Autodesk Inventor part; units mm, degrees
ref_plane "YZ Plane" through (0, 0, 0) normal (1, 0, 0) x (0, 1, 0)
ref_plane "XZ Plane" through (0, 0, 0) normal (0, 1, 0) x (-1, 0, 0)
ref_plane "XY Plane" through (0, 0, 0) normal (0, 0, 1) x (1, 0, 0)
sketch "Sketch1" plane through (0, 0, 0) normal (0, 1, 0) x (-1, 0, 0)
  line L0 (0, 0) -> (115, 0)
  line L1 (115, 0) -> (115, -215)
  line L2 (115, -215) -> (0, -215)
  line L3 (0, -215) -> (0, 0)
  dimension "d0" = 115
  dimension "d1" = 215
extrude "Extrusion1" add sketch "Sketch1" along normal blind 50
sketch "Sketch2" plane through (-115, 0, 0) normal (0, 0, 1) x (1, 0, 0)
  line L0 (115, 0) -> (115, 5)
  line L1 (115, 0) -> (115, 50)
  line L2 (115, 5) -> (43, 5)
  line L3 (43, 5) -> (43, 17)
  line L4 (43, 17) -> (115, 17)
  line L5 (115, 17) -> (115, 5)
  dimension "d4" = 5
  dimension "d5" = 72
  dimension "d6" = 12
extrude "Extrusion2" add sketch "Sketch2" along normal blind 12
properties part number "S-201-24"
Verification items for the finished model (mm, model axes). A direction names the side the tool comes from. Round coordinates to 2 decimals unless told otherwise and drop trailing zeros. Order: outer loops, then holes, each group sorted by start corner. A loop starts at its lowest first (then second) coordinate and runs counter-clockwise, first axis right, second up.
1. Section check D-D on y = 32.5. Record the cut outline in (x, z).
Final values:
outline: (-115, -215) - (0, -215) - (0, 0) - (-115, 0) - close
2. Section check A-A on x = -22.5. Record the cut outline in (y, z), then the cut area to 3 significant figures.
Final values:
outline: (0, -215) - (50, -215) - (50, 0) - (17, 0) - (17, 12) - (5, 12) - (5, 0) - (0, 0) - close
area: 10,900 mm2
3. Release check for a two-part mould opening along Z. For faces 4 (the flat face through (-35, 5, 6)), 5 (the flat face through (-37, 11, 12)), 6 (the flat face through (-58, 25, -215)) record: +Z half, -Z half, draft (parallel to the pull), parting line (faces both ways), or undercut.
Final values:
face 4: draft
face 5: +Z half
face 6: -Z half
4. Go/stop test with flat-tipped pins: P1, Ø9.5, axis at y = 11.5, z = 6.5, coming from the -X side; P2, Ø6, axis at x = -45, z = 4, coming from the +Y side; P3, Ø13, axis at x = -53.5, z = 7.5, coming from the -Y side. Record where each tip stops, or that it passes through.
Final values:
P1: stops at x = -72
P2: stops at y = 17
P3: stops at y = 5
5. Section check C-C on x = -89.5. Record the cut outline in (y, z).
Final values:
outline: (0, -215) - (50, -215) - (50, 0) - (0, 0) - close
6. Thickness scan on L1, parallel to Z at x = -75.5, y = 7. Record the ranges inside material, lowest first.
Final values:
L1: z = -215 to 0
7. Access from +Z, -Z, +X, -X, +Y, -Y to the whole of each face (thin tool, end or side, straight path). Record for faces 1 (the flat face through (-37, 17, 6)), 2 (the flat face through (-72, 11, 6)), 3 (the flat face through (0, 25, -103)).
Final values:
face 1: +Z, +X, -X, +Y
face 2: +Z, -X, +Y, -Y
face 3: +Z, -Z, +X, +Y, -Y
8. Section check B-B on y = 14. Record the cut outline in (x, z), then the cut area to 3 significant figures.
Final values:
outline: (-115, -215) - (0, -215) - (0, 12) - (-72, 12) - (-72, 0) - (-115, 0) - close
area: 25,600 mm2
